The model under review builds one solid part; all positions refer to its coordinate system, in mm. A direction names the side the tool comes from. Coordinates: 2 decimals unless noted, no trailing zeros. Write each loop counter-clockwise with the first axis right and the second up, starting at its lowest first coordinate (ties: lowest second). Pieces come first, ordered by that corner, then holes.
```python
from build123d import *

# Parameters (mm, degrees)
BOSS_EXTRUDE1_DEPTH = 2
BOSS_EXTRUDE2_DEPTH = 3
SKETCH3_W           = 7
SKETCH3_H           = 3.108863517
BOSS_EXTRUDE3_DEPTH = 2


with BuildPart() as part:
    # Sketch1 → Boss-Extrude1 (new body)
    with BuildSketch(Plane(origin=(0, 0, 0), x_dir=(1, 0, 0), z_dir=(0, 1, 0))):
        Polygon((-7.5, -4.5), (7.5, -4.5), (11.4, -4.5), (11.4, 4.5), (7.5, 4.5), (-7.5, 4.5), (-7.5, 5.5), (-14.5, 5.5), (-14.5, -5.5), (-7.5, -5.5), align=None)
    extrude(amount=BOSS_EXTRUDE1_DEPTH)

    # Sketch2 → Boss-Extrude2 (add)
    with BuildSketch(Plane(origin=(0, 0, 0), x_dir=(1, 0, 0), z_dir=(0, 1, 0))):
        Polygon((7.5, 4.5), (-7.5, 4.5), (-7.5, 5.5), (-14.5, 5.5), (-14.5, 3.5), (0.5, 3.5), (0.5, 3), (7.5, 3), (9.9, 3), (9.9, -4.5), (11.4, -4.5), (11.4, 4.5), align=None)
        Polygon((-7.5, -4.5), (-7.5, -5.5), (-14.5, -5.5), (-14.5, -3.5), (0.5, -3.5), (0.5, -3), (5.986157355, -3), (5.986157355, -4.5), align=None)
        Polygon((0.5, 1.6), (7.5, 1.6), (8.5, 1.6), (8.5, -4.5), (7.5, -4.5), (7.5, -1.6), (0.5, -1.6), align=None)
    extrude(amount=-BOSS_EXTRUDE2_DEPTH)

    # Sketch3 → Boss-Extrude3 (add)
    with BuildSketch(Plane.XZ.offset(3)):
        with Locations((-11, 3.945568242)):
            Rectangle(SKETCH3_W, SKETCH3_H)
        with Locations((-11, -3.945568242)):
            Rectangle(SKETCH3_W, SKETCH3_H)
    extrude(amount=-BOSS_EXTRUDE3_DEPTH)


solid = part.part
```
Item 1: For pin 1 (1.5 mm diameter, centred on x = 6, y = -0.5, fed in from -Z); pin 2 (1 mm diameter, centred on x = -6.5, y = -1, fed in from +Z); pin 3 (3 mm diameter, centred on x = -7.5, z = -2, fed in from -Y); pin 4 (2.5 mm diameter, centred on y = -1.5, z = 0, fed in from -X), all flat-tipped, find the tip position at first contact; note any pin that passes through.
Solved:
pin 1: stops at z = -4.5
pin 2: stops at z = 4.5
pin 3: stops at y = -3
pin 4: stops at x = 0.5
Item 2: Machinability: for faces 4 (the face through (5, -1, -1.6)), 5 (the face through (5.986, -1, 4)), 6 (the face through (2, 0, 4.5)), which of the approach directions +Z, -Z, +X, -X, +Y, -Y give a long, thin tool a straight path to every point of the face, cutting with its end or side? Answer none if there is none.
Solved:
face 4: -X, -Y
face 5: +Z, -Y
face 6: +Z, +X, +Y, -Y
Item 3: Take a section at B-B, the plane x = 4. Write out the cut boundary in (y, z).
Solved:
outline: (-3, -4.5) - (2, -4.5) - (2, 4.5) - (-3, 4.5) - (-3, 3) - (0, 3) - (0, 1.6) - (-3, 1.6) - (-3, -1.6) - (0, -1.6) - (0, -3) - (-3, -3) - close
Item 4: Take a section at D-D, the plane z = 0. Write out the cut boundary in (x, y).
Solved:
outline: (-14.5, 0) - (0.5, 0) - (0.5, -3) - (8.5, -3) - (8.5, 0) - (9.9, 0) - (9.9, -3) - (11.4, -3) - (11.4, 2) - (-14.5, 2) - close
Item 5: Take a section at C-C, the plane y = 1.3. Write out the cut boundary in (x, z).
Solved:
outline: (-14.5, -5.5) - (-7.5, -5.5) - (-7.5, -4.5) - (11.4, -4.5) - (11.4, 4.5) - (-7.5, 4.5) - (-7.5, 5.5) - (-14.5, 5.5) - close
Item 6: Mouldability with a two-part tool opening along Y and no side actions: class faces 1 (the face through (-11, -1, 3)), 2 (the face through (7.5, -1, 3)), 3 (the face through (0, -3, -4)) as pulls with the +Y half, pulls with the -Y half, needs draft (parallel to the pull), parting line crosses it, or undercut.
Solved:
face 1: undercut
face 2: needs draft
face 3: pulls with the -Y half
Item 7: Take a section at A-A, the plane y = -0.25. Write out the cut boundary in (x, z), plus the area to 3 significant figures.
Solved:
outline: (-14.5, -5.5) - (-7.5, -5.5) - (-7.5, -4.5) - (11.4, -4.5) - (11.4, 4.5) - (9.9, 4.5) - (9.9, -3) - (0.5, -3) - (0.5, -3.5) - (-14.5, -3.5) - close; (-14.5, 3.5) - (0.5, 3.5) - (0.5, 3) - (5.99, 3) - (5.99, 4.5) - (-7.5, 4.5) - (-7.5, 5.5) - (-14.5, 5.5) - close; (0.5, -1.6) - (8.5, -1.6) - (8.5, 4.5) - (7.5, 4.5) - (7.5, 1.6) - (0.5, 1.6) - close
area: 108 mm2
Item 8: To check wall thickness, follow line 1 along Z through (x, y) = (1.5, -0.8); line 2 along X through (y, z) = (-1.2, 1.75); line 3 along X through (y, z) = (-0.9, 0.5). State the ranges of each line that lie inside material, in increasing order.
Solved:
line 1: z = -4.5 to -3, -1.6 to 1.6, 3 to 4.5
line 2: x = 7.5 to 8.5, 9.9 to 11.4
line 3: x = 0.5 to 8.5, 9.9 to 11.4
